```python
from build123d import *

# Parameters (mm, degrees)
BOX001_W       = 10
BOX001_H       = 10
BOX001_DEPTH   = 8
CYLINDER_R     = 1.5
CYLINDER_DEPTH = 5
BOX_W          = 16
BOX_H          = 16
BOX_DEPTH      = 10


with BuildPart() as cube001:
    # Box001 → Box001 (new body)
    with BuildSketch(Plane(origin=(-5, -5, 0), x_dir=(1, 0, 0), z_dir=(0, 0, 1))):
        with Locations((5, 5)):
            Rectangle(BOX001_W, BOX001_H)
    extrude(amount=BOX001_DEPTH)


with BuildPart() as cylinder:
    # Cylinder → Cylinder (new body)
    with BuildSketch(Plane.XY.offset(10)):
        Circle(CYLINDER_R)
    extrude(amount=CYLINDER_DEPTH)


with BuildPart() as sphere:
    # Sphere → Sphere (revolve)
    with BuildSketch(Plane(origin=(0, 0, 17), x_dir=(1, 0, 0), z_dir=(0, -1, 0))):
        with BuildLine():
            ThreePointArc((0, -3), (3, 0), (0, 3))
            Line((0, 3), (0, -3))
        make_face()
    revolve(axis=Axis((0, 0, 17), (0, 0, 1)))


with BuildPart() as cut:
    # Box → Box (new body)
    with BuildSketch(Plane(origin=(-8, -8, 0), x_dir=(1, 0, 0), z_dir=(0, 0, 1))):
        with Locations((8, 8)):
            Rectangle(BOX_W, BOX_H)
    extrude(amount=BOX_DEPTH)

    # Fusion: union Cylinder, Sphere
    add(cylinder.part)
    add(sphere.part)

    # Cut: cut Cube001
    add(cube001.part, mode=Mode.SUBTRACT)


solid = cut.part
```
Geometry check sheet. Reference: the model listing, model coordinates, mm. A direction names the side the tool comes from. Coordinates: 2 decimals unless noted, no trailing zeros. Loops run counter-clockwise (first coordinate to the right, second up) from the corner with the lowest first, then second, coordinate; pieces in that order, holes last.
Item 1: Thickness scan on line 1 (X direction, y = -3.25, z = 7.75); line 2 (Z direction, x = -6.5, y = -1). Record the ranges inside material, lowest first.
Item 2: Go/stop test with flat-tipped pins: pin 1 Ø3 at (x, y) = (-1, 0.5) entering from -Z; pin 2 Ø4 at (y, z) = (2.5, 17) entering from +X. Record where each tip stops, or that it passes through.
Item 3: Sectioned sample at A-A, the plane y = 4.5. Record the boundary of the cut face in (x, z), then the cut area to 3 significant figures.
Item 4: Sectioned sample at B-B, the plane x = -2.5. Record the boundary of the cut face in (y, z).
Item 5: Access from +Z, -Z, +X, -X, +Y, -Y to the whole of each face (thin tool, end or side, straight path). Record for faces 1 (the face through (0, 0, 8)), 2 (the face through (8, 0, 5)), 3 (the face through (-1.5, 0.07, 12.17)).
Item 6: Release check for a two-part mould opening along Y. For faces 4 (the face through (0, -8, 5)), 5 (the face through (0, 2, 10)), 6 (the face through (0, 5, 4)) record: released by +Y, released by -Y, zero draft, split by the parting line, or undercut.
Item 7: Sectioned sample at D-D, the plane x = 0. Record the boundary of the cut face in (y, z).
Item 8: Sectioned sample at C-C, the plane y = -2. Record the boundary of the cut face in (x, z).
Check result:
1. line 1: x = -8 to -5, 5 to 8
1. line 2: z = 0 to 10
2. pin 1: stops at z = 8
2. pin 2: stops at x = 2.96
3. outline: (-8, 0) - (-5, 0) - (-5, 8) - (5, 8) - (5, 0) - (8, 0) - (8, 10) - (-8, 10) - close
3. area: 80.0 mm2
4. outline: (-8, 0) - (-5, 0) - (-5, 8) - (5, 8) - (5, 0) - (8, 0) - (8, 10) - (-8, 10) - close; circle Ø3.32 at (0, 17)
5. face 1: -Z
5. face 2: +Z, -Z, +X, +Y, -Y
5. face 3: none
6. face 4: released by -Y
6. face 5: zero draft
6. face 6: undercut
7. outline: (-8, 0) - (-5, 0) - (-5, 8) - (5, 8) - (5, 0) - (8, 0) - (8, 10) - (1.5, 10) - (1.5, 14.4) arc R3 ccw (long way) to (-1.5, 14.4) - (-1.5, 10) - (-8, 10) - close
8. outline: (-8, 0) - (-5, 0) - (-5, 8) - (5, 8) - (5, 0) - (8, 0) - (8, 10) - (-8, 10) - close; circle Ø4.47 at (0, 17)
